from build123d import *

# Parameters (mm, degrees)
SKETCH1_R           = 12.7
BOSS_EXTRUDE1_DEPTH = 75
SKETCH5_R           = 12.7
CUT_EXTRUDE1_DEPTH  = 37.5
SKETCH2_R           = 10
BOSS_EXTRUDE2_DEPTH = 40


with BuildPart() as part:
    # Sketch1 → Boss-Extrude1 (new body)
    with BuildSketch(Plane(origin=(0, 0, 0), x_dir=(0, 0, -1), z_dir=(1, 0, 0))):
        Circle(SKETCH1_R)
    extrude(amount=BOSS_EXTRUDE1_DEPTH)

    # Sketch5 → Cut-Extrude1 (cut, symmetric)
    with BuildSketch(Plane(origin=(0, 0, 0), x_dir=(1, 0, 0), z_dir=(0, 1, 0))):
        Circle(SKETCH5_R)
    extrude(amount=CUT_EXTRUDE1_DEPTH, both=True, mode=Mode.SUBTRACT)

    # Sketch2 → Boss-Extrude2 (add)
    with BuildSketch(Plane(origin=(75, 0, 0), x_dir=(0, 0, -1), z_dir=(1, 0, 0))):
        Circle(SKETCH2_R)
    extrude(amount=BOSS_EXTRUDE2_DEPTH)


solid = part.part
Geometry: final body of the model. Coordinates: model frame, mm. A direction names the side the tool comes from. Give positions to 0.01 mm unless a question says otherwise; leave off trailing zeros. Write each loop counter-clockwise with the first axis right and the second up, starting at its lowest first coordinate (ties: lowest second). Pieces come first, ordered by that corner, then holes. Notation, with made-up numbers: (53.25, 4.25) -> (92.25, 4.25) arc R26 cw to (92.25, 24.25) -> close; hole circle Ø4 at (80, -0.75). An arc over 180 degrees is marked (long way). Answer in a Markdown table with one row per item.
(1) Section query C-C on x = 87. Return loops of the section in (y, z), then the cut area to 3 significant figures.
Answers below:
| item | result |
|---|---|
| outline | circle Ø20 at (0, 0) |
| area | 314 mm^2 |
(2) Section query A-A on y = 0. Return loops of the section in (x, z).
Answers below:
| item | result |
|---|---|
| outline | (0, -12.7) -> (75, -12.7) -> (75, -10) -> (115, -10) -> (115, 10) -> (75, 10) -> (75, 12.7) -> (0, 12.7) arc R12.7 cw to start |
(3) Section query B-B on z = 0. Return loops of the section in (x, y), then the cut area to 3 significant figures.
Answers below:
| item | result |
|---|---|
| outline | (12.7, -12.7) -> (75, -12.7) -> (75, -10) -> (115, -10) -> (115, 10) -> (75, 10) -> (75, 12.7) -> (12.7, 12.7) -> close |
| area | 2,380 mm^2 |
(4) Section query D-D on x = 60.5. Return loops of the section in (y, z).
Answers below:
| item | result |
|---|---|
| outline | circle Ø25.4 at (0, 0) |
(5) Pin query (flat end, axial travel): pin 1 (8 mm diameter, centred on x = 54.5, y = -7, fed in from -Z); pin 2 (4 mm diameter, centred on x = 101, z = -5, fed in from -Y); pin 3 (3 mm diameter, centred on x = 74, y = 5.5, fed in from +Z). Return the tip coordinate at first contact, or that it passes through.
Answers below:
| item | result |
|---|---|
| pin 1 | z = -12.34 |
| pin 2 | y = -9.54 |
| pin 3 | z = 12.05 |
(6) Ray query, line 1 along X through (y, z) = (10.25, 0.25); line 2 along Z through (x, y) = (55.5, 0.5); line 3 along X through (y, z) = (9.5, 7). Return the intervals inside material, ascending. Write a range as [from, to].
Answers below:
| item | result |
|---|---|
| line 1 | [12.7, 75] |
| line 2 | [-12.69, 12.69] |
| line 3 | [10.6, 75] |
(7) Set-up query: faces 4 (the flat face through (115, 0, 0)), 5 (the cylindrical face through (94.72, -9.76, 2.17)). Return all of +Z, -Z, +X, -X, +Y, -Y with unobstructed straight access to the full face (end or side cutting, diameter ignored); none if empty.
Answers below:
| item | result |
|---|---|
| face 4 | +Z, -Z, +X, +Y, -Y |
| face 5 | +X |
(8) Draft query along Z for faces 1 (the flat face through (75, -10.3, 0.1)), 2 (the cylindrical face through (45.308, 0.558, 12.688)), 3 (the cylindrical face through (12.697, 0.178, 0.279)). Return one class per face: +Z half, -Z half, draft (parallel to the pull), parting line (faces both ways), or undercut.
Answers below:
| item | result |
|---|---|
| face 1 | draft |
| face 2 | parting line |
| face 3 | undercut |
